For this review, use the dimensioned drawing (mm, ordinates from the lowest corner) and the shaded views. Give positions to 0.01 mm unless a question says otherwise; leave off trailing zeros. Loops run counter-clockwise (first coordinate to the right, second up) from the corner with the lowest first, then second, coordinate; pieces in that order, holes last. Notation, with made-up numbers: M 1,46 L 30,46 A18 ccw 30,52 Z; hole C -17.5,86.25 d11. An arc over 180 degrees is marked long. Return JSON: item names as keys, results as strings.
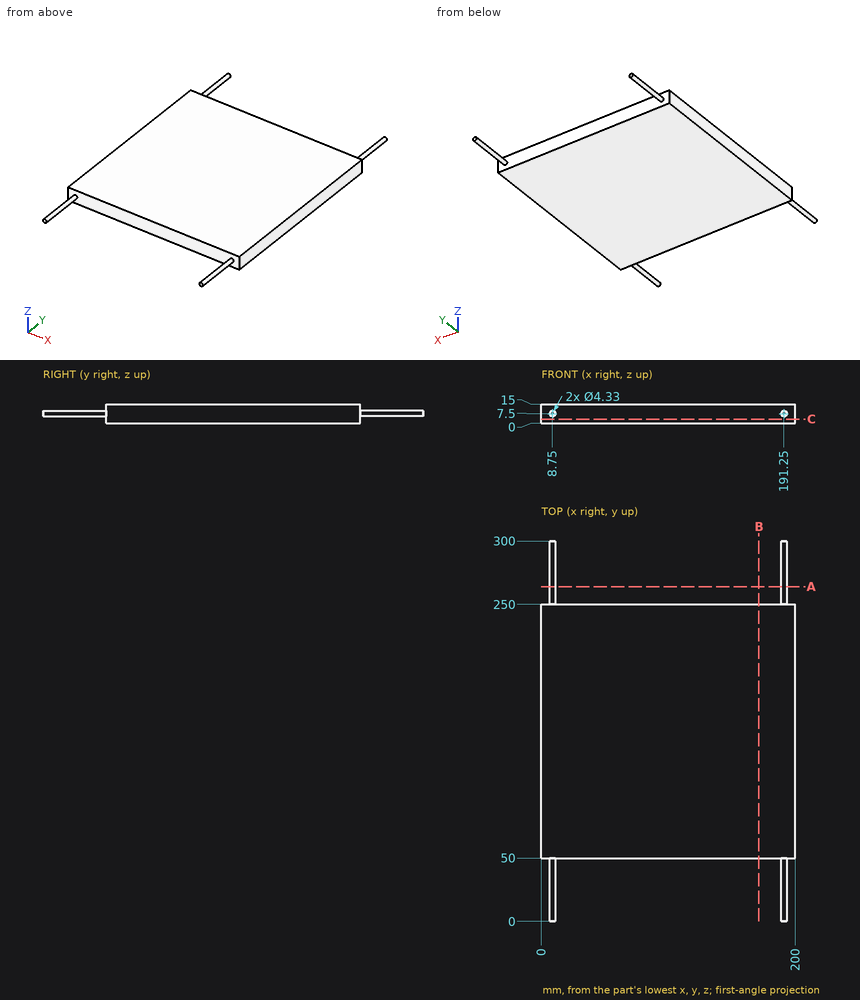
1) Consider section C-C on z = 3. Write out the cut boundary in (x, y).
From the geometry:
{"outline": "M 0,50 L 200,50 L 200,250 L 0,250 Z"}
2) Insertion check: pin 1 (12 mm diameter, centred on x = 171, y = 63, fed in from -Z); pin 2 (4.5 mm diameter, centred on x = 51.5, z = 10, fed in from -Y). Each pin has a flat end and moves straight along its axis. Give the tip position at first contact, or say it passes through.
From the geometry:
{"pin 1": "z = 0", "pin 2": "y = 50"}
3) Consider section B-B on x = 171.5. Write out the cut boundary in (y, z), then the cut area to 3 significant figures.
From the geometry:
{"outline": "M 50,0 L 250,0 L 250,15 L 50,15 Z", "area": "3,000 mm²"}
4) Wall thickness on L1, parallel to X at y = 264.5, z = 8; L2, parallel to Y at x = 121, z = 11.75; L3, parallel to X at y = 15, z = 9.25: over which ranges is each line inside the solid? List them lowest first. Write a range as from..to.
From the geometry:
{"L1": "6.64..10.86, 189.14..193.36", "L2": "50..250", "L3": "7.48..10.02, 189.98..192.52"}
5) Consider section A-A on y = 264. Write out the cut boundary in (x, z) (3 decimals).
From the geometry:
{"outline": "C 8.75,7.5 d4.33; C 191.25,7.5 d4.33"}
